from build123d import *

# Parameters (mm, degrees)
SCHIZZO2_W                   = 4.6
SCHIZZO2_H                   = 1
ESTRUSIONE_ESTRUSIONE1_DEPTH = 8


with BuildPart() as part:
    # Schizzo1 → Rivoluzione1 (revolve)
    with BuildSketch(Plane(origin=(0, 0, 0), x_dir=(0, 0, -1), z_dir=(1, 0, 0)), mode=Mode.PRIVATE) as rivoluzione1_sk:
        Polygon((-17, 6.5), (-16.35, 7.15), (-14.2, 7.15), (-14.2, 6), (1.5, 6), (2, 5), (7, 5), (7, 0), (0, 0), (0, 3), (-17, 3), (-17, 4), (0, 4), (0, 5), (-17, 5), align=None)
    revolve(rivoluzione1_sk.sketch.rotate(Axis((0, 0, 0), (0, 0, -1)), 90), axis=Axis((0, 0, 0), (0, 0, -1)))

    # Schizzo2 → Estrusione-Estrusione1 (add)
    with BuildSketch(Plane(origin=(0, 0, -7), x_dir=(-1, 0, 0), z_dir=(0, 0, -1))):
        Rectangle(SCHIZZO2_W, SCHIZZO2_H)
    extrude(amount=ESTRUSIONE_ESTRUSIONE1_DEPTH)


solid = part.part
Could you check a few things on this model? Use its own coordinates, in mm. A direction names the side the tool comes from. Give positions to 0.01 mm unless a question says otherwise; leave off trailing zeros. Order: outer loops, then holes, each group sorted by start corner. A loop starts at its lowest first (then second) coordinate and runs counter-clockwise, first axis right, second up.
1. We'd pull the mould along Y, two halves only. Please class faces 1 (the flat face through (-1, -3, 17)), 2 (the flat face through (0, -0.5, -11)), 3 (the cylindrical face through (-5, 0, 9)), 4 (the cylindrical face through (-0.867, 3.905, 8.381)): pulls with the +Y half, pulls with the -Y half, needs draft (parallel to the pull), parting line crosses it, or undercut.
2. Will these pins go through, and if not, where does the flat tip stop? P1, Ø1.4, axis at x = -1, z = -9, coming from the +Y side; P2, Ø2, axis at x = 4.5, y = 2, coming from the -Z side; P3, Ø1.1, axis at y = 0, z = -12, coming from the +X side.
3. Suppose I cut it at D-D (z = -6). List the corners of the cut face in (x, y) for me, plus the area to 3 significant figures.
4. I need wall thicknesses on L1, parallel to Y at x = 0, z = 13; L2, parallel to Z at x = -1, y = -6.25; L3, parallel to Y at x = -0.75, z = 10. Which ranges of each line are inside material? Lowest first, please.
5. Suppose I cut it at A-A (z = 0.5). List the corners of the cut face in (x, y) for me.
6. For faces 5 (the flat face through (-2, -6, 14.2)), 6 (the cylindrical face through (2.86, -0.9, 8.62)), 7 (the flat face through (0, 0.5, -11)), which set-ups out of +Z, -Z, +X, -X, +Y, -Y let a thin tool reach every point of the face, with its end or its side?
Solved:
1. face 1: needs draft
1. face 2: pulls with the -Y half
1. face 3: undercut
1. face 4: undercut
2. P1: stops at y = 0.5
2. P2: stops at z = -7
2. P3: stops at x = 2.3
3. outline: circle Ø10 at (0, 0)
3. area: 78.5 mm2
4. L1: y = -6 to -5, -4 to -3, 3 to 4, 5 to 6
4. L2: z = 14.2 to 17
4. L3: y = -5.95 to -4.94, -3.93 to -2.9, 2.9 to 3.93, 4.94 to 5.95
5. outline: circle Ø12 at (0, 0); circle Ø8 at (0, 0); hole circle Ø10 at (0, 0); hole circle Ø6 at (0, 0)
6. face 5: -Z
6. face 6: +Z
6. face 7: -Z, +X, -X, +Y
